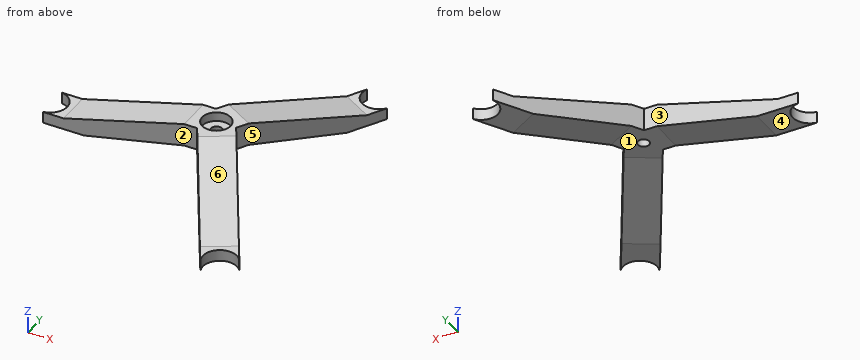
from build123d import *

# Parameters (mm, degrees)
F1_DEPTH  = 9.525
F3_DEPTH  = 6.351
F0_W      = 12.7
F0_H      = 12.7
F4_DEPTH  = 9.525
F6_DEPTH  = 5.08
F8_DEPTH  = 25.4
F10_COUNT = 3


with BuildPart() as f1:
    # F0 (on Front) → F1 (new body, symmetric)
    with BuildSketch(Plane.XZ):
        Polygon((-91.44, 0), (-68.58, 0), (-68.58, 6.35), (-80.01, 6.35), (-91.44, 6.35), align=None)
        Polygon((-68.58, 6.35), (-68.58, 0), (-12.7, 12.621443), (-12.7, 25.321443), (-80.01, 6.35), align=None)
    extrude(amount=F1_DEPTH, both=True)

    # F2 (on face) → F3 (cut, through all)
    with BuildSketch(Plane.XY.offset(6.35)):
        with BuildLine():
            Line((-91.44, 9.439954), (-91.44, -9.439954))
            ThreePointArc((-91.44, -9.439954), (-83.185, 0), (-91.44, 9.439954))
        make_face()
    extrude(amount=-F3_DEPTH, mode=Mode.SUBTRACT)

    # F0 (on Front) → F4 (join, symmetric)
    with BuildSketch(Plane.XZ):
        with Locations((-6.35, 18.971443)):
            Rectangle(F0_W, F0_H)
    extrude(amount=F4_DEPTH, both=True)

    # F5 (on face) → F6 (cut)
    with BuildSketch(Plane.XY.offset(25.321443)):
        with BuildLine():
            Line((0, -7.9375), (0, 7.9375))
            ThreePointArc((0, 7.9375), (-7.9375, 0), (0, -7.9375))
        make_face()
    extrude(amount=-F6_DEPTH, mode=Mode.SUBTRACT)

    # F7 (on face) → F8 (cut)
    with BuildSketch(Plane.XY.offset(20.241443)):
        with BuildLine():
            Line((0, -3.175), (0, 3.175))
            ThreePointArc((0, 3.175), (-3.175, 0), (0, -3.175))
        make_face()
    extrude(amount=-F8_DEPTH, mode=Mode.SUBTRACT)

    # F10: F1 ×3 about axis
    f10_axis = Axis((0, 0, 19.108918), (0, 0, 1))


with BuildPart() as f1_1:
    add(f1.part)
    for i in range(1, F10_COUNT):
        add(f1.part.rotate(f10_axis, i * 360 / F10_COUNT))


solid = f1_1.part
The listing builds one solid part. Answer for the finished solid, in the listing's coordinates (mm). Face numbers are marked on the shaded views. A direction names the side the tool comes from. Give positions to 0.01 mm unless a question says otherwise; leave off trailing zeros. Loops run counter-clockwise (first coordinate to the right, second up) from the corner with the lowest first, then second, coordinate; pieces in that order, holes last.
Item 1: A tool of negligible diameter and unlimited length cuts with its end or side. For the marked faces 1, 2 and 3, from which of +Z, -Z, +X, -X, +Y, -Y can it reach the whole face along a straight path? Write none if from no direction.
Derived:
face 1: -Z
face 2: +Z, -Z, -X, -Y
face 3: +Z, -Z, -X, +Y
Item 2: Determine the mould class of the marked faces 4, 5 and 6 for opening direction Y: +Y half, -Y half, draft (parallel to the pull), parting line (faces both ways), or undercut.
Derived:
face 4: draft
face 5: undercut
face 6: -Y half
Item 3: Each of these flat-tipped pins is pushed along its axis until it touches: pin 1 Ø12.5 at (x, z) = (-67.5, 12) entering from +Y (3 decimals); pin 2 Ø1 at (y, z) = (-29.5, 8.5) entering from +X; pin 3 Ø13.5 at (x, y) = (-5, 0.5) entering from -Z. Where does it stop, or does it pass through?
Derived:
pin 1: stops at y = 9.525
pin 2: stops at x = 28.32
pin 3: stops at z = 12.62
Item 4: Find the intervals of material crossed by line 1 along Y through (x, z) = (20.5, 11.5); line 2 along Y through (x, z) = (0, 14.5) (3 decimals); line 3 along X through (y, z) = (-28, 9.5), in increasing order.
Derived:
line 1: y = -54.56 to -16.46, 16.46 to 54.56
line 2: y = -19.05 to -3.175, 3.175 to 19.05
line 3: x = 5.17 to 27.16
Item 5: A cutting plane is placed at C-C (y = -50.5). Give the vertices of the cut face in (x, z), then the cut area to 3 significant figures.
Derived:
outline: (18.16, 3.56) - (40.15, 1.08) - (40.15, 10.92) - (18.16, 14.02) - close
area: 223 mm2
Item 6: A cutting plane is placed at D-D (x = -75.5). Give the vertices of the cut face in (y, z) (3 decimals), then the cut area to 3 significant figures.
Derived:
outline: (-9.525, 0) - (9.525, 0) - (9.525, 7.621) - (-9.525, 7.621) - close
area: 145 mm2
Item 7: A cutting plane is placed at A-A (z = 14.75). Give the vertices of the cut face in (x, y) (3 decimals), then the cut area to 3 significant figures.
Derived:
outline: (-50.207, -9.525) - (-5.499, -9.525) - (16.855, -48.243) - (33.352, -38.718) - (10.999, 0) - (33.352, 38.718) - (16.855, 48.243) - (-5.499, 9.525) - (-50.207, 9.525) - close; hole circle Ø6.35 at (0, 0)
area: 2,680 mm2
